For this review, take the finished solid that the model builds, in its own axes (mm). Round coordinates to 2 decimals unless told otherwise and drop trailing zeros. Write each loop counter-clockwise with the first axis right and the second up, starting at its lowest first coordinate (ties: lowest second). Pieces come first, ordered by that corner, then holes.
from build123d import *

# Parameters (mm, degrees)
F1_DEPTH = 19.05
F3_DEPTH = 19.05


with BuildPart() as f1:
    # F0 (on Front) → F1 (new body)
    with BuildSketch(Plane.XZ):
        with BuildLine():
            Line((119.888, 155.774192), (0, 155.774192))
            Line((0, 155.774192), (-119.888, 155.774192))
            Line((-119.888, 155.774192), (-119.888, 143.074192))
            Line((-119.888, 143.074192), (-247.076714, -163.503496))
            Line((-247.076714, -163.503496), (-119.888, -163.503496))
            ThreePointArc((-119.888, -163.503496), (0, 1.376312), (119.888, -163.503496))
            Line((119.888, -163.503496), (247.076714, -163.503496))
            Line((247.076714, -163.503496), (119.888, 143.074192))
            Line((119.888, 143.074192), (119.888, 155.774192))
        make_face()
    extrude(amount=F1_DEPTH)

    # F2 (on Front) → F3 (cut)
    with BuildSketch(Plane.XZ):
        Polygon((-9.779, 105.583792), (0, 105.583792), (9.779, 105.583792), (9.779, 155.774192), (0, 155.774192), (-9.779, 155.774192), align=None)
    extrude(amount=F3_DEPTH, mode=Mode.SUBTRACT)


solid = f1.part
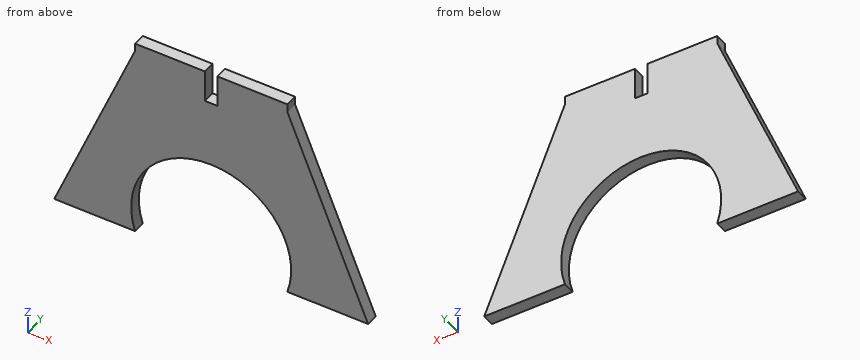
(1) We need section A-A, the plane z = -112. Give the boundary of the cut face in (x, y).
Geometry check:
outline: (-225.71, -19.05) - (-125.39, -19.05) - (-125.39, 0) - (-225.71, 0) - close; (125.39, -19.05) - (225.71, -19.05) - (225.71, 0) - (125.39, 0) - close
(2) We need section C-C, the plane x = 0. Give the boundary of the cut face in (y, z), and give its area (3 significant figures).
Geometry check:
outline: (-19.05, 1.38) - (0, 1.38) - (0, 105.58) - (-19.05, 105.58) - close
area: 1,990 mm2
(3) For line 1 along Z through (x, y) = (0, -9); line 2 along X through (y, z) = (-10.25, -100.5); line 3 along X through (y, z) = (-10.5, -97), list the stretches that pass through material, from the lowest coordinate up.
Geometry check:
line 1: z = 1.38 to 105.58
line 2: x = -220.94 to -123.69, 123.69 to 220.94
line 3: x = -219.49 to -122.96, 122.96 to 219.49
(4) We need section D-D, the plane z = -45. Give the boundary of the cut face in (x, y), and give its area (3 significant figures).
Geometry check:
outline: (-197.91, -19.05) - (-97.67, -19.05) - (-97.67, 0) - (-197.91, 0) - close; (97.67, -19.05) - (197.91, -19.05) - (197.91, 0) - (97.67, 0) - close
area: 3,820 mm2
(5) We need section B-B, the plane y = -5.5. Give the boundary of the cut face in (x, z), and give its area (3 significant figures).
Geometry check:
outline: (-247.08, -163.5) - (-119.89, -163.5) arc R126.03 cw (long way) to (119.89, -163.5) - (247.08, -163.5) - (119.89, 143.07) - (119.89, 155.77) - (9.78, 155.77) - (9.78, 105.58) - (-9.78, 105.58) - (-9.78, 155.77) - (-119.89, 155.77) - (-119.89, 143.07) - close
area: 80,000 mm2
(6) For pin 1 Ø9.5 at (y, z) = (-5.5, 121.5) entering from +X; pin 2 Ø4 at (x, y) = (-45.5, -7.5) entering from -Z; pin 3 Ø5.5 at (x, y) = (4, -9.5) entering from +Z; pin 4 Ø8 at (x, z) = (-143.5, 44.5) entering from +Y, all flat-tipped, find the tip position at first contact; note any pin that passes through.
Geometry check:
pin 1: stops at x = 130.81
pin 2: stops at z = -7.92
pin 3: stops at z = 105.58
pin 4: stops at y = 0
